Part model, mm, in its own coordinate system. Coordinates: 2 decimals unless noted, no trailing zeros. Loops run counter-clockwise (first coordinate to the right, second up) from the corner with the lowest first, then second, coordinate; pieces in that order, holes last. Notation, with made-up numbers: M 73,77 L 94,77 A32 cw 94,113 Z; hole C 16.25,58.25 d3. An arc over 180 degrees is marked long. Use CSV: the item, a comma, the result in double quotes. Start each with the question number.
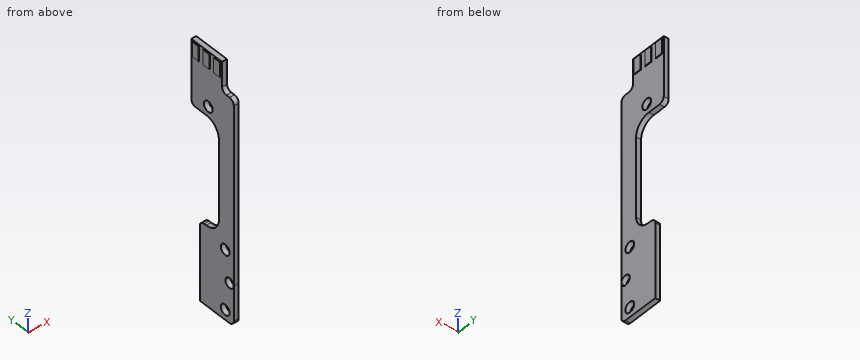
Autodesk Inventor part; units mm, degrees
ref_plane "YZ Plane" through (0, 0, 0) normal (1, 0, 0) x (0, 1, 0)
ref_plane "XZ Plane" through (0, 0, 0) normal (0, 1, 0) x (-1, 0, 0)
ref_plane "XY Plane" through (0, 0, 0) normal (0, 0, 1) x (1, 0, 0)
sketch "Skizze1" plane through (0, 0, 0) normal (1, 0, 0) x (0, 1, 0)
  line L0 (0, 0) -> (8, 0)
  line L1 (8, 0) -> (8, 16)
  line L2 (8, 16) -> (3.5, 16)
  line L3 (0, 51) -> (0, 0)
  circle A0 centre (1, 8) radius 1
  circle A1 centre (2, 14) radius 1.05
  circle A2 centre (2, 2) radius 1.05
  line L4 (2, 14) -> (2, 2) construction
  line L5 (2, 8) -> (1, 8) construction
  line L6 (3.5, 16) -> (3.5, 38)
  line L7 (3.5, 38) -> (10, 38)
  line L8 (10, 38) -> (10, 51)
  line L9 (10, 51) -> (0, 51)
  dimension "d1" = 16
  dimension "d2" = 2
  dimension "d3" = 1
  dimension "d4" = 8
  dimension "d5" = 2.1
  dimension "d6" = 2.1
  dimension "d14" = 12
  dimension "d15" = 1
  dimension "d28" = 8
  dimension "d29" = 3.5
  dimension "d30" = 35
  dimension "d31" = 10
  dimension "d32" = 13
extrude "Extrusion1" add sketch "Skizze1" along normal blind 1
sketch "Skizze2" plane through (0, 0, 0) normal (-1, 0, 0) x (0, 0, 1)
  circle A0 centre (2, 2) radius 1.05
  circle A1 centre (14, 2) radius 1.05
  line L0 (0, 0) -> (0, 8)
  line L1 (8, 0) -> (0, 0)
  circle A2 centre (8, 1) radius 1
  line L2 (51, 0) -> (8, 0)
  line L3 (16, 8) -> (16, 3.5)
  line L4 (0, 8) -> (16, 8)
  line L5 (50.7, 3.15) -> (47.7, 3.15)
  line L6 (47.7, 3.15) -> (47.7, 4.65)
  line L7 (47.7, 4.65) -> (50.7, 4.65)
  line L8 (50.7, 4.65) -> (50.7, 3.15)
  line L9 (50.7, 5.65) -> (47.7, 5.65)
  line L10 (47.7, 5.65) -> (47.7, 7.15)
  line L11 (47.7, 7.15) -> (50.7, 7.15)
  line L12 (50.7, 7.15) -> (50.7, 5.65)
  line L13 (50.7, 8.15) -> (47.7, 8.15)
  line L14 (47.7, 8.15) -> (47.7, 9.65)
  line L15 (47.7, 9.65) -> (50.7, 9.65)
  line L16 (50.7, 9.65) -> (50.7, 8.15)
  line L17 (51, 10) -> (51, 0)
  line L18 (38, 10) -> (51, 10)
  line L19 (38, 3.5) -> (38, 10)
  line L20 (16, 3.5) -> (38, 3.5)
  line L21 (50.7, 3.9) -> (47.7, 3.9) construction
  line L22 (47.7, 6.4) -> (50.7, 6.4) construction
  line L23 (50.7, 8.9) -> (47.7, 8.9) construction
  dimension "d16" = 1.5
  dimension "d17" = 1.5
  dimension "d21" = 3
  dimension "d26" = 1.5
  dimension "d34" = 2.5
  dimension "d35" = 2.5
  dimension "d36" = 0.3
  dimension "d37" = 6.4
extrude "Extrusion2" add sketch "Skizze2" along normal blind 0.1 and the other way blind 1.1 contours L5 L6 L7 L8 | L9 L10 L11 L12 | L13 L14 L15 L16
fillet "Rundung1" radius 3 2 edges at (0.5, 3.5, 16) (0.5, 3.5, 38)
sketch "Skizze3" plane through (0, 0, 51) normal (-1, 0, 0) x (0, 0, 1)
  circle A0 centre (-43, 1) radius 1
  point P0 (-51, 0)
  point P1 (-11, 6)
  point P2 (-43, 0)
  dimension "d38" = 5
  dimension "d39" = 32
hole "Bohrung1" at (0, 6, 40) direction (1, 0, 0) diameter 2.1 end through all
fillet "Rundung2" radius 1 2 edges at (0.5, 10, 38) (0.5, 8, 16)
fillet "Rundung3" radius 1 1 edges at (0.5, 0, 0)
sketch "Skizze4" plane through (1, 1, 8) normal (1, 0, 0) x (0, 0, -1)
  line L0 (-43, -1) -> (0, -1)
  line L1 (-43, 9) -> (-43, -1)
  line L2 (-43, -1) -> (-37, -1)
  line L3 (-37, -1) -> (-37, 1.75)
  line L4 (-37, 1.75) -> (-43, 1.75)
  line L5 (-43, 1.75) -> (-43, -1)
  point P0 (8, -1)
  dimension "d52" = 2.75
  dimension "d53" = 6
extrude "Extrusion3" cut sketch "Skizze4" against normal through all
fillet "Rundung4" radius 1 2 edges at (0.5, 2.75, 45) (0.5, 0, 45)
properties part number "IR Platine" material "Phenolharz"
1. Pin check, flat tips, straight feed: pin 1 (1.5 mm diameter, centred on y = 5.5, z = 12.5, fed in from +X); pin 2 (3.5 mm diameter, centred on y = 2, z = 14, fed in from -X). Stop position of each tip, or through.
2. Slice it at D-D, the plane z = 29.5. List the corners of the cut face in (x, y).
3. Wall check: probe 1 along Y at (x, z) = (0.8, 40); probe 2 along Z at (x, y) = (0.9, 1.75); probe 3 along X at (y, z) = (6, 42). Give the ranges that are in metal, low to high.
4. Slice it at C-C, the plane z = 40. List the corners of the cut face in (x, y), and give its area (3 significant figures).
5. Slice it at A-A, the plane z = 14. List the corners of the cut face in (x, y), and give its area (3 significant figures).
Found:
1,pin 1,"x = 1"
1,pin 2,"x = 0"
2,outline,"M 0,0 L 1,0 L 1,3.5 L 0,3.5 Z"
3,probe 1,"0 to 4.95, 7.05 to 10"
3,probe 2,"0 to 0.98, 3.02 to 7.34, 8.66 to 12.98, 15.02 to 45"
3,probe 3,"0 to 1"
4,outline,"M 0,0 L 1,0 L 1,4.95 L 0,4.95 Z; M 0,7.05 L 1,7.05 L 1,10 L 0,10 Z"
4,area,"7.90 mm^2"
5,outline,"M 0,0 L 1,0 L 1,0.95 L 0,0.95 Z; M 0,3.05 L 1,3.05 L 1,8 L 0,8 Z"
5,area,"5.90 mm^2"
